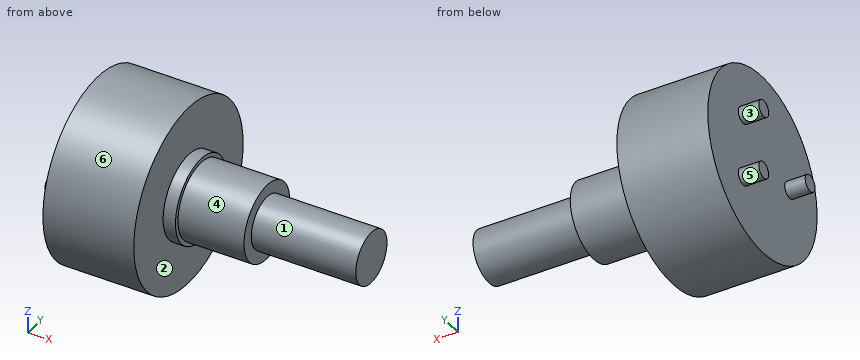
from build123d import *

# Parameters (mm, degrees)
SKETCH2_R           = 1
BOSS_EXTRUDE1_DEPTH = 2.49


with BuildPart() as part:
    # Sketch1 → Revolve1 (revolve)
    with BuildSketch(Plane.XY):
        Polygon((-16.64, 0), (16.64, 0), (16.64, 3.175), (3.94, 3.175), (3.94, 4.655), (-4.09, 4.655), (-4.09, 5.155), (-5.59, 5.155), (-5.59, 11.115), (-16.64, 11.115), align=None)
    revolve(axis=Axis((-16.64, 0, 0), (1, 0, 0)))

    # Sketch2 → Boss-Extrude1 (add)
    with BuildSketch(Plane.ZY.offset(16.64)):
        with Locations((-3.905, 3.908529135)):
            Circle(SKETCH2_R)
        with Locations((3.905, 3.908529135)):
            Circle(SKETCH2_R)
        with Locations((0, -5.525)):
            Circle(SKETCH2_R)
    extrude(amount=BOSS_EXTRUDE1_DEPTH)


solid = part.part
Geometry check sheet. Reference: the model listing, model coordinates, mm. Face numbers are marked on the shaded views. A direction names the side the tool comes from. Give positions to 0.01 mm unless a question says otherwise; leave off trailing zeros. Loops run counter-clockwise (first coordinate to the right, second up) from the corner with the lowest first, then second, coordinate; pieces in that order, holes last. Notation, with made-up numbers: M 85.25,-6 L 93.25,-6 A16 ccw 93.25,9 Z; hole C -27,-19.75 d2. An arc over 180 degrees is marked long. Answer as a JSON object with one key per item and string values. Group by question number.
Item 1: Mould release check, pull along Z, two halves, no side actions. Record for the marked faces 1, 2 and 3: pulls with the +Z half, pulls with the -Z half, needs draft (parallel to the pull), parting line crosses it, or undercut.
Item 2: Sectioned sample at C-C on x = 9. Record the boundary of the cut face in (y, z) (3 decimals), plus the area to 3 significant figures.
Item 3: Sectioned sample at B-B on z = 0. Record the boundary of the cut face in (x, y) (3 decimals).
Item 4: Material ranges on L1, parallel to X at y = 8, z = 3.5; L2, parallel to X at y = -1, z = 2.75; L3, parallel to Z at x = -11, y = 8.75, recorded low to high.
Item 5: Sectioned sample at D-D on y = -2.5. Record the boundary of the cut face in (x, z).
Item 6: Gauge pin test, flat ends, axial feed: pin 1 (4 mm diameter, centred on y = -2.5, z = 6.5, fed in from -X); pin 2 (2 mm diameter, centred on x = -12, z = -3, fed in from +Y); pin 3 (3 mm diameter, centred on y = 3.5, z = 7.5, fed in from +X). Record the tip position at first contact, or that the pin passes through.
Item 7: Sectioned sample at A-A on y = 0.75. Record the boundary of the cut face in (x, z).
Item 8: Access from +Z, -Z, +X, -X, +Y, -Y to the whole of each face (thin tool, end or side, straight path). Record for the marked faces 4, 5 and 6.
Findings below:
{
 "1": {"face 1": "parting line crosses it", "face 2": "needs draft", "face 3": "undercut"},
 "2": {"outline": "C 0,0 d6.35", "area": "31.7 mm2"},
 "3": {"outline": "M -19.13,-6.525 L -16.64,-6.525 L -16.64,-11.115 L -5.59,-11.115 L -5.59,-5.155 L -4.09,-5.155 L -4.09,-4.655 L 3.94,-4.655 L 3.94,-3.175 L 16.64,-3.175 L 16.64,3.175 L 3.94,3.175 L 3.94,4.655 L -4.09,4.655 L -4.09,5.155 L -5.59,5.155 L -5.59,11.115 L -16.64,11.115 L -16.64,-4.525 L -19.13,-4.525 Z"},
 "4": {"L1": "-16.64 to -5.59", "L2": "-16.64 to 16.64", "L3": "-6.85 to 6.85"},
 "5": {"outline": "M -16.64,-10.83 L -5.59,-10.83 L -5.59,-4.51 L -4.09,-4.51 L -4.09,-3.93 L 3.94,-3.93 L 3.94,-1.96 L 16.64,-1.96 L 16.64,1.96 L 3.94,1.96 L 3.94,3.93 L -4.09,3.93 L -4.09,4.51 L -5.59,4.51 L -5.59,10.83 L -16.64,10.83 Z"},
 "6": {"pin 1": "x = -16.64", "pin 2": "y = 10.93", "pin 3": "x = -5.59"},
 "7": {"outline": "M -16.64,-11.09 L -5.59,-11.09 L -5.59,-5.1 L -4.09,-5.1 L -4.09,-4.59 L 3.94,-4.59 L 3.94,-3.09 L 16.64,-3.09 L 16.64,3.09 L 3.94,3.09 L 3.94,4.59 L -4.09,4.59 L -4.09,5.1 L -5.59,5.1 L -5.59,11.09 L -16.64,11.09 Z"},
 "8": {"face 4": "+X", "face 5": "-X", "face 6": "+X, -X"}
}
